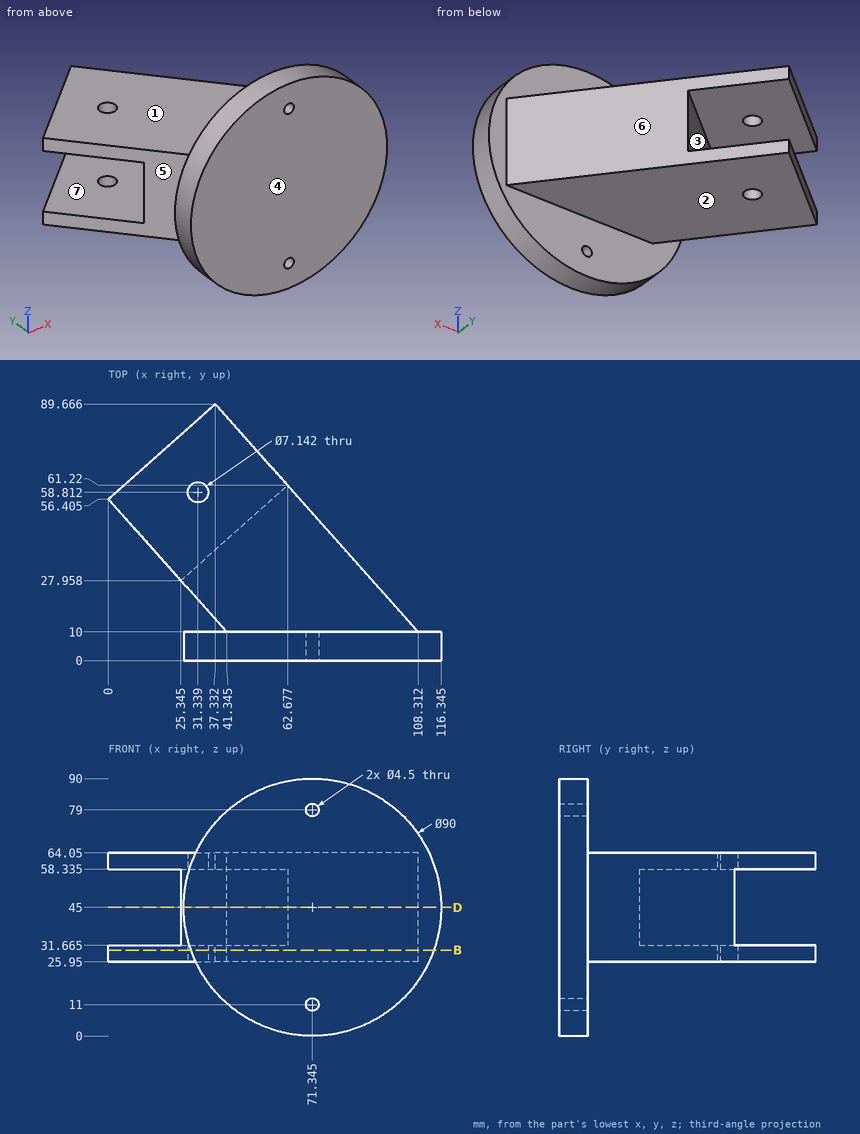
Can you work these out from the drawing? Everything is in mm from the part's minimum corner. A direction names the side the tool comes from. Round coordinates to 2 decimals unless told otherwise and drop trailing zeros. Write each loop counter-clockwise with the first axis right and the second up, starting at its lowest first coordinate (ties: lowest second). Pieces come first, ordered by that corner, then holes. Notation, with made-up numbers: (38, 57) - (87, 57) arc R35 ccw to (87, 91) - close; hole circle Ø7 at (43, 56). An arc over 180 degrees is marked (long way). Write each question's results on one line, items separated by ' | '. Start each with the question number.
1) Please list where these lines run through material, in increasing order: line 1 (Z direction, x = 82, y = 29); line 2 (Y direction, x = 32.5, z = 23).
2) Suppose I cut it at D-D (z = 45). List the corners of the cut face in (x, y) for me (1 decimal), and give its area (3 significant figures).
3) For pin 1 Ø2.5 at (x, z) = (71.35, 79) entering from +Y; pin 2 Ø5 at (x, y) = (62.5, 43) entering from -Z; pin 3 Ø24 at (x, y) = (65, 59) entering from +Z; pin 4 Ø12 at (x, z) = (91.5, 35) entering from +Y (1 decimal), each with a flat end and sliding along its axis, tell me the tip position at first contact or that it passes through.
4) Which directions (+Z, -Z, +X, -X, +Y, -Y) give clear straight access to the entire face, cutting with the end or side of a thin tool? Please do the marked faces 1, 2 and 3.
5) We'd pull the mould along Y, two halves only. Please class the marked faces 4, 5, 6 and 7: released by +Y, released by -Y, zero draft, split by the parting line, or undercut.
6) Suppose I cut it at B-B (z = 30). List the corners of the cut face in (x, y) for me (1 decimal), and give its area (3 significant figures).
Here are the results:
1) line 1: z = 25.95 to 64.05 | line 2: y = 0 to 10
2) outline: (25.3, 28) - (41.3, 10) - (26.3, 10) - (26.3, 0) - (116.3, 0) - (116.3, 10) - (108.3, 10) - (62.7, 61.2) - close | area: 3,220 mm2
3) pin 1: passes through | pin 2: stops at z = 25.95 | pin 3: stops at z = 64.05 | pin 4: stops at y = 35.6
4) face 1: +Z, +X, -X, +Y | face 2: -Z, +X, -X, +Y | face 3: -X, +Y
5) face 4: released by -Y | face 5: undercut | face 6: released by +Y | face 7: zero draft
6) outline: (0, 56.4) - (41.3, 10) - (28.9, 10) - (28.9, 0) - (113.8, 0) - (113.8, 10) - (108.3, 10) - (37.3, 89.7) - close; hole circle Ø7.1 at (31.3, 58.8) | area: 5,030 mm2
